Model file for the job. Use its own axes, mm. Round coordinates to 2 decimals unless told otherwise and drop trailing zeros. Order: outer loops, then holes, each group sorted by start corner. A loop starts at its lowest first (then second) coordinate and runs counter-clockwise, first axis right, second up. Notation, with made-up numbers: M 44.5,-30 L 103.5,-30 A22 ccw 103.5,-11 Z; hole C 75.5,9 d2. An arc over 180 degrees is marked long. Return JSON: item names as keys, results as strings. Group by question number.
Item 1: Pin check, flat tip, straight feed: pin 1 Ø2 at (x, z) = (-1.5, 81.5) entering from +Y. Stop position of the tip, or through.
Item 2: Slice it at C-C on z = 299.5. Write the cut outline in (x, y), then the cut area to 3 significant figures.
Item 3: Slice it at A-A on x = 0. Write the cut outline in (y, z), then the cut area to 3 significant figures.
Item 4: Probe line 1 along Z through (x, y) = (-0.5, 3); line 2 along Z through (x, y) = (-0.75, -2.25); line 3 along Y through (x, z) = (-0.5, 24). List the from-to ranges inside material, lowest first.
from build123d import *

# Parameters (mm, degrees)
SKETCH1_R           = 2.5
EXTRUDE1_DEPTH      = 40
SKETCH2_R           = 4
BOSS_EXTRUDE1_DEPTH = 302
FILLET1_R           = 0.25


with BuildPart() as part:
    # Sketch1 → Extrude1 (new body)
    with BuildSketch(Plane.XY):
        Circle(SKETCH1_R)
    extrude(amount=EXTRUDE1_DEPTH)

    # Sketch2 → Boss-Extrude1 (add)
    with BuildSketch(Plane.XY.offset(40)):
        Circle(SKETCH2_R)
    extrude(amount=BOSS_EXTRUDE1_DEPTH)

    # Fillet1
    fillet1_edges = [part.edges().sort_by_distance(p)[0] for p in [
        (-2.5, 0, 0),
        (-4, 0, 342),
    ]]
    fillet(fillet1_edges, radius=FILLET1_R)


solid = part.part
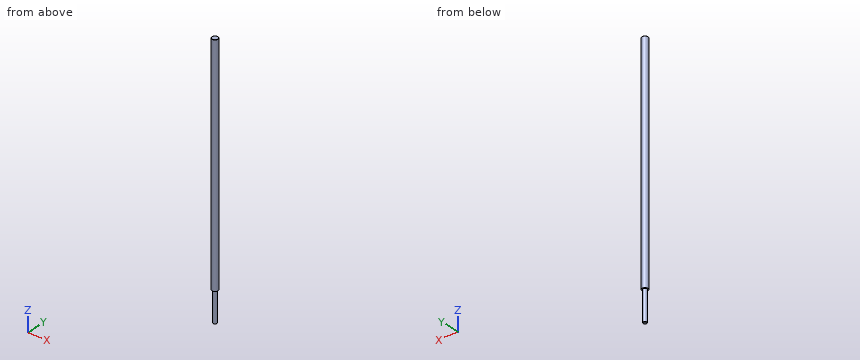
Output values:
{
 "1": {"pin 1": "y = 3.97"},
 "2": {"outline": "C 0,0 d8", "area": "50.3 mm²"},
 "3": {"outline": "M -4,40 L -2.5,40 L -2.5,0.25 A0.25 ccw -2.25,0 L 2.25,0 A0.25 ccw 2.5,0.25 L 2.5,40 L 4,40 L 4,341.75 A0.25 ccw 3.75,342 L -3.75,342 A0.25 ccw -4,341.75 Z", "area": "2,620 mm²"},
 "4": {"line 1": "40 to 342", "line 2": "0.03 to 342", "line 3": "-2.45 to 2.45"}
}
